Verification items for the finished model (mm, model axes). Face numbers are marked on the shaded views. A direction names the side the tool comes from. Coordinates: 2 decimals unless noted, no trailing zeros. Order: outer loops, then holes, each group sorted by start corner. A loop starts at its lowest first (then second) coordinate and runs counter-clockwise, first axis right, second up. Notation, with made-up numbers: (-11, 8.5) - (36, 8.5) arc R21 ccw to (36, 44.5) - close; hole circle Ø4 at (20, 72.25). An arc over 180 degrees is marked (long way). Answer as CSV lines item,"result". Start each with the question number.
1. Set-up check for the marked faces 3 and 4: record each of +Z, -Z, +X, -X, +Y, -Y from which the full face is reachable in a straight line by a thin tool's end or side.
2. Section check A-A (x = 0). Record the cut outline in (y, z), and give its area (3 significant figures).
3. Mould release check, pull along Y, two halves, no side actions. Record for the marked faces 1 and 2: pulls with the +Y half, pulls with the -Y half, needs draft (parallel to the pull), parting line crosses it, or undercut.
4. Section check C-C (z = 1884.5). Record the cut outline in (x, y), and give its area (3 significant figures).
5. Section check D-D (x = 198.5). Record the cut outline in (y, z), and give its area (3 significant figures).
6. Material ranges on L1, parallel to Z at x = 90, y = -219.5; L2, parallel to Y at x = 0, z = 1502; L3, parallel to Y at x = 0, z = 2268.5, recorded low to high. Write a range as [from, to].
7. Go/stop test with flat-tipped pins: pin 1 (1 mm diameter, centred on y = 39.5, z = 1396, fed in from -X); pin 2 (6 mm diameter, centred on x = 39.5, y = 76.5, fed in from +Z); pin 3 (2 mm diameter, centred on x = 117.5, z = 1357, fed in from +Y). Record where each tip stops, or that it passes through.
8. Section check B-B (y = -142.5). Record the cut outline in (x, z), and give its area (3 significant figures).
from build123d import *

# Parameters (mm, degrees)
SKETCH1_R           = 250
BOSS_EXTRUDE1_DEPTH = 2198
SHELL2_T            = -2
SKETCH2_R           = 100
SKETCH2_R_2         = 98
EXTRUDE_THIN1_DEPTH = 150
SKETCH3_R           = 250
SKETCH3_R_2         = 98
BOSS_EXTRUDE2_DEPTH = 1


with BuildPart() as part:
    # Sketch1 → Boss-Extrude1 (new body)
    with BuildSketch(Plane.XY):
        Circle(SKETCH1_R)
    extrude(amount=BOSS_EXTRUDE1_DEPTH)

    # Shell2
    shell2_openings = [part.faces().sort_by_distance(p)[0] for p in [
        (0, 0, 2198),
    ]]
    offset(amount=SHELL2_T, openings=shell2_openings, kind=Kind.INTERSECTION)



with BuildPart() as body_2:
    # Sketch2 → Extrude-Thin1 (new body)
    with BuildSketch(Plane.XY.offset(2198)):
        Circle(SKETCH2_R)
        Circle(SKETCH2_R_2, mode=Mode.SUBTRACT)
    extrude(amount=EXTRUDE_THIN1_DEPTH)


with BuildPart() as part_1:
    add(part.part)

    add(body_2.part)  # Boss-Extrude2 merges body 2
    # Sketch3 → Boss-Extrude2 (add)
    with BuildSketch(Plane.XY.offset(2198)):
        Circle(SKETCH3_R)
        Circle(SKETCH3_R_2, mode=Mode.SUBTRACT)
    extrude(amount=BOSS_EXTRUDE2_DEPTH)


solid = part_1.part
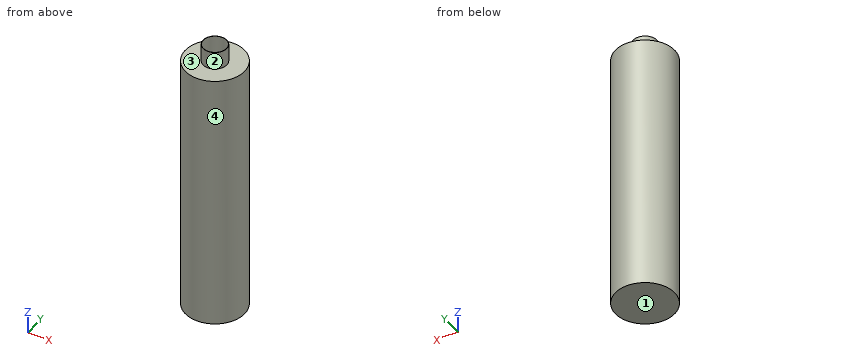
Evaluation:
1,face 3,"+Z"
1,face 4,"+Z, -Z"
2,outline,"(-250, 0) - (250, 0) - (250, 2199) - (100, 2199) - (100, 2348) - (98, 2348) - (98, 2198) - (248, 2198) - (248, 2) - (-248, 2) - (-248, 2198) - (-98, 2198) - (-98, 2348) - (-100, 2348) - (-100, 2199) - (-250, 2199) - close"
2,area,"10,700 mm²"
3,face 1,"needs draft"
3,face 2,"parting line crosses it"
4,outline,"circle Ø500 at (0, 0); hole circle Ø496 at (0, 0)"
4,area,"3,130 mm²"
5,outline,"(-151.98, 0) - (151.98, 0) - (151.98, 2199) - (-151.98, 2199) - close; hole (-148.67, 2) - (148.67, 2) - (148.67, 2198) - (-148.67, 2198) - close"
5,area,"15,500 mm²"
6,L1,"z = [0, 2], [2198, 2199]"
6,L2,"y = [-250, -248], [248, 250]"
6,L3,"y = [-100, -98], [98, 100]"
7,pin 1,"stops at x = -246.94"
7,pin 2,"stops at z = 2"
7,pin 3,"stops at y = 221.2"
8,outline,"(-205.41, 0) - (205.41, 0) - (205.41, 2199) - (-205.41, 2199) - close; hole (-202.97, 2) - (202.97, 2) - (202.97, 2198) - (-202.97, 2198) - close"
8,area,"11,900 mm²"
